from build123d import *

# Parameters (mm, degrees)
SKETCH_1_R          = 5.5
SKETCH_1_R_2        = 2
EXTRUDE_1_DEPTH     = 4
SKETCH_2_R          = 5.2
SKETCH_2_R_2        = 2.7
CUT_EXTRUDE_1_DEPTH = 0.2
CUT_EXTRUDE_START   = -3.8
SKETCH_2_2_R        = 5.2
SKETCH_2_2_R_2      = 2.7
CUT_EXTRUDE_2_DEPTH = 5.946427842
CHAMFER_1_SIZE      = 0.05


with BuildPart() as part:
    # Sketch 1 → Extrude 1 (new body)
    with BuildSketch(Plane(origin=(0, 0, 0), x_dir=(1, 0, 0), z_dir=(0, 1, 0))):
        with Locations(Location((0, 0, 0), (0, 0, 270))):
            Circle(SKETCH_1_R)
        with Locations(Location((0, 0, 0), (0, 0, 270))):
            Circle(SKETCH_1_R_2, mode=Mode.SUBTRACT)
    extrude(amount=EXTRUDE_1_DEPTH)

    # Sketch 2 → Cut-Extrude 1 (cut)
    with BuildSketch(Plane(origin=(0, 4, 0), x_dir=(1, 0, 0), z_dir=(0, 1, 0))):
        with Locations(Location((0, 0, 0), (0, 0, 270))):
            Circle(SKETCH_2_R)
        with Locations(Location((0, 0, 0), (0, 0, 270))):
            Circle(SKETCH_2_R_2, mode=Mode.SUBTRACT)
    extrude(amount=-CUT_EXTRUDE_1_DEPTH, mode=Mode.SUBTRACT)

    # Sketch 2_2 → Cut-Extrude 2 (cut, through all)
    with BuildSketch(Plane(origin=(0, 4, 0), x_dir=(1, 0, 0), z_dir=(0, 1, 0)).offset(CUT_EXTRUDE_START)):
        with Locations(Location((0, 0, 0), (0, 0, 270))):
            Circle(SKETCH_2_2_R)
        with Locations(Location((0, 0, 0), (0, 0, 270))):
            Circle(SKETCH_2_2_R_2, mode=Mode.SUBTRACT)
    extrude(amount=-CUT_EXTRUDE_2_DEPTH, mode=Mode.SUBTRACT)

    # Chamfer 1
    chamfer_1_edges = [part.edges().sort_by_distance(p)[0] for p in [
        (0, 4, -5.2),
        (0, 4, -2.7),
        (0, 0, -5.2),
        (0, 0, -2.7),
        (0, 0, -5.5),
        (0, 4, -5.5),
        (0, 0, -2),
        (0, 4, -2),
    ]]
    chamfer(chamfer_1_edges, length=CHAMFER_1_SIZE)


solid = part.part
The listing builds one solid part. Answer for the finished solid, in the listing's coordinates (mm). A direction names the side the tool comes from. Round coordinates to 2 decimals unless told otherwise and drop trailing zeros. Order: outer loops, then holes, each group sorted by start corner. A loop starts at its lowest first (then second) coordinate and runs counter-clockwise, first axis right, second up. Notation, with made-up numbers: M -40,88.5 L 5,88.5 A16 cw 5,116.5 Z; hole C 58.25,-22.5 d2. An arc over 180 degrees is marked long. Answer in a Markdown table with one row per item. Add a question column.
1) The part is cut by section A-A on y = 3.55. Determine the outline of the cut face in (x, z), plus the area to 3 significant figures.
2) Which of the six approach directions +Z, -Z, +X, -X, +Y, -Y give full straight-line access (tool end or side, diameter ignored) to faces 1 (the face through (-2.2, 0.2, 2.2)), 2 (the face through (-2.2, 3.8, 2.2)), 3 (the face through (-2, 4, 1))?
3) Determine the mould class of faces 4 (the face through (-2, 0, 1)), 5 (the face through (-2, 2, 0)) for opening direction Z: pulls with the +Z half, pulls with the -Z half, needs draft (parallel to the pull), parting line crosses it, or undercut.
4) A flat-ended cylindrical pin translates along its axis: pin 1 Ø3 at (x, z) = (0, 0) entering from +Y. Find the tip coordinate at first contact, or state that the pin passes through.
5) Consider line 1 along X through (y, z) = (3.85, 0); line 2 along X through (y, z) = (1.9, 0); line 3 along Y through (x, z) = (2.5, 4). Determine where each line is inside the solid, lowest interval first. Write a range as from..to.
Findings below:
| question | item | result |
|---|---|---|
| 1 | outline | C 0,0 d11; hole C 0,0 d4 |
| 1 | area | 82.5 mm² |
| 2 | face 1 | -Y |
| 2 | face 2 | +Y |
| 2 | face 3 | +Z, -Z, +X, -X, +Y |
| 3 | face 4 | needs draft |
| 3 | face 5 | undercut |
| 4 | pin 1 | passes through |
| 5 | line 1 | x = -5.5..-5.2, -2.7..-2, 2..2.7, 5.2..5.5 |
| 5 | line 2 | x = -5.5..-2, 2..5.5 |
| 5 | line 3 | y = 0.2..3.8 |
